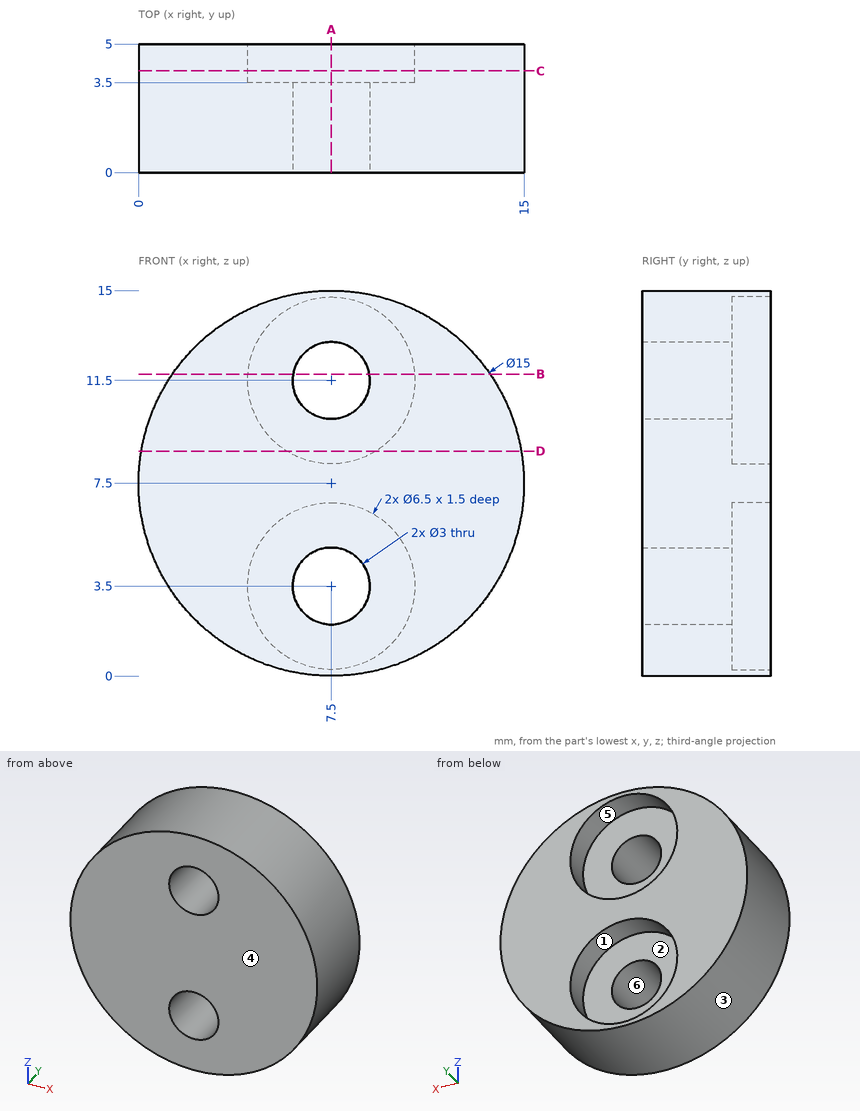
Print and shaded views of the part. All mm, measured from the part's lowest x, y and z. A direction names the side the tool comes from. Give positions to 0.01 mm unless a question says otherwise; leave off trailing zeros. Write each loop counter-clockwise with the first axis right and the second up, starting at its lowest first coordinate (ties: lowest second). Pieces come first, ordered by that corner, then holes. Notation, with made-up numbers: (-31.5, 38.5) - (1.5, 38.5) arc R24 ccw to (1.5, 59.5) - close; hole circle Ø11 at (77.25, 27.25). An arc over 180 degrees is marked (long way). One line per question, with ' | ' between items. Start each with the question number.
(1) Slice it at D-D on z = 8.75. Write the cut outline in (x, y), plus the area to 3 significant figures.
(2) Slice it at A-A on x = 7.5. Write the cut outline in (y, z).
(3) Two-plate mould, pull along Z, no slides. Class the marked faces 1, 2, 3 and 4: +Z half, -Z half, draft (parallel to the pull), parting line (faces both ways), or undercut.
(4) Slice it at B-B on z = 11.75. Write the cut outline in (x, y), plus the area to 3 significant figures.
(5) Pin check, flat tips, straight feed: P1, Ø3, axis at x = 7.5, z = 4.5, coming from the +Y side; P2, Ø2, axis at x = 11.5, y = 1.5, coming from the -Z side; P3, Ø2, axis at y = 3.5, z = 12.5, coming from the -X side. Stop position of each tip, or through.
(6) Slice it at C-C on y = 3.95. Write the cut outline in (x, z), plus the area to 3 significant figures.
(7) 3-axis set-ups, long thin cutter, end or side, ignore diameter. For the marked faces 5 and 6: which of +Z, -Z, +X, -X, +Y, -Y reach the whole face in a straight line?
(8) Wall check: line 1 along Z through (x, y) = (8.5, 3.75); line 2 along Z through (x, y) = (6.25, 3); line 3 along X through (y, z) = (4.3, 7.25). Give the ranges that are in metal, low to high. Write a range as from..to.
Results below:
1) outline: (0.1, 0) - (14.9, 0) - (14.9, 5) - (9.23, 5) - (9.23, 3.5) - (5.77, 3.5) - (5.77, 5) - (0.1, 5) - close | area: 68.8 mm^2
2) outline: (0, 0) - (5, 0) - (5, 0.25) - (3.5, 0.25) - (3.5, 2) - (0, 2) - close; (0, 5) - (3.5, 5) - (3.5, 6.75) - (5, 6.75) - (5, 8.25) - (3.5, 8.25) - (3.5, 10) - (0, 10) - close; (0, 13) - (3.5, 13) - (3.5, 14.75) - (5, 14.75) - (5, 15) - (0, 15) - close
3) face 1: undercut | face 2: undercut | face 3: parting line | face 4: draft
4) outline: (1.32, 0) - (6.02, 0) - (6.02, 3.5) - (4.26, 3.5) - (4.26, 5) - (1.32, 5) - close; (8.98, 0) - (13.68, 0) - (13.68, 5) - (10.74, 5) - (10.74, 3.5) - (8.98, 3.5) - close | area: 41.7 mm^2
5) P1: y = 3.5 | P2: z = 0.63 | P3: x = 1.16
6) outline: circle Ø15 at (7.5, 7.5); hole circle Ø6.5 at (7.5, 3.5); hole circle Ø6.5 at (7.5, 11.5) | area: 110 mm^2
7) face 5: +Y | face 6: +Y, -Y
8) line 1: 0.07..0.41, 6.59..8.41, 14.59..14.93 | line 2: 0.1..2.67, 4.33..10.67, 12.33..14.9 | line 3: 0..15
